```python
from build123d import *

# Parameters (mm, degrees)
SALIENTE_EXTRUIR1_DEPTH = 10
CROQUIS2_R              = 2.5
CORTAR_EXTRUIR1_DEPTH   = 1.5
CROQUIS3_R              = 1.5
CORTAR_EXTRUIR2_DEPTH   = 2
CORTAR_EXTRUIR3_START   = -24
CROQUIS6_R              = 1
CORTAR_EXTRUIR3_DEPTH   = 24
CROQUIS9_W              = 7
CROQUIS9_H              = 5
CROQUIS9_R              = 0.5
SALIENTE_EXTRUIR4_DEPTH = 6
CROQUIS10_W             = 3
CROQUIS10_H             = 3
CORTAR_EXTRUIR4_DEPTH   = 5
REDONDEO1_R             = 5


with BuildPart() as part:
    # Croquis1 → Saliente-Extruir1 (new body)
    with BuildSketch(Plane.XY):
        Polygon((8.5, 0), (-8.5, 0), (-8.5, -12.5), (-12, -12.5), (-12, 2.5), (-12, 15), (-9.5, 15), (-9.5, 2.5), (9.5, 2.5), (9.5, 15), (12, 15), (12, 2.5), (12, -12.5), (8.5, -12.5), align=None)
    extrude(amount=SALIENTE_EXTRUIR1_DEPTH)

    # Croquis2 → Cortar-Extruir1 (cut)
    with BuildSketch(Plane(origin=(-8.5, 0, 0), x_dir=(0, 0, -1), z_dir=(1, 0, 0))):
        with Locations(Location((-5, -8.5, 0), (0, 0, 90))):
            Circle(CROQUIS2_R)
    cortar_extruir1 = extrude(amount=-CORTAR_EXTRUIR1_DEPTH, mode=Mode.SUBTRACT)

    # Croquis3 → Cortar-Extruir2 (cut)
    with BuildSketch(Plane(origin=(-10, 0, 0), x_dir=(0, 0, -1), z_dir=(1, 0, 0))):
        with Locations(Location((-5, -8.5, 0), (0, 0, 90))):
            Circle(CROQUIS3_R)
    cortar_extruir2 = extrude(amount=-CORTAR_EXTRUIR2_DEPTH, mode=Mode.SUBTRACT)

    # Simetría1: Cortar-Extruir1, Cortar-Extruir2 across plane
    add(cortar_extruir1.mirror(Plane(origin=(0, 0, 0), x_dir=(0, 0, 1), z_dir=(1, 0, 0))), mode=Mode.SUBTRACT)
    add(cortar_extruir2.mirror(Plane(origin=(0, 0, 0), x_dir=(0, 0, 1), z_dir=(1, 0, 0))), mode=Mode.SUBTRACT)

    # Croquis6 → Cortar-Extruir3 (cut)
    with BuildSketch(Plane.ZY.offset(12).offset(CORTAR_EXTRUIR3_START)):
        with Locations((5, 12)):
            Circle(CROQUIS6_R)
    extrude(amount=CORTAR_EXTRUIR3_DEPTH, mode=Mode.SUBTRACT)

    # Croquis9 → Saliente-Extruir4 (add)
    with BuildSketch(Plane.ZY.offset(12)):
        with Locations((6.5, 7)):
            Rectangle(CROQUIS9_W, CROQUIS9_H)
        with Locations((5, 7)):
            Circle(CROQUIS9_R, mode=Mode.SUBTRACT)
    extrude(amount=SALIENTE_EXTRUIR4_DEPTH)

    # Croquis10 → Cortar-Extruir4 (cut)
    with BuildSketch(Plane.XZ.offset(-4.5)):
        with Locations((-13.5, 4.5)):
            Rectangle(CROQUIS10_W, CROQUIS10_H)
    extrude(amount=-CORTAR_EXTRUIR4_DEPTH, mode=Mode.SUBTRACT)

    # Redondeo1
    redondeo1_edges = [part.edges().sort_by_distance(p)[0] for p in [
        (10.25, -12.5, 10),
        (-10.25, -12.5, 10),
        (-10.25, -12.5, 0),
        (10.25, -12.5, 0),
        (-10.75, 15, 10),
        (-10.75, 15, 0),
        (10.75, 15, 10),
        (10.75, 15, 0),
    ]]
    fillet(redondeo1_edges, radius=REDONDEO1_R - 0.0001)  # a hair under: the kernel refuses the full size


solid = part.part
```
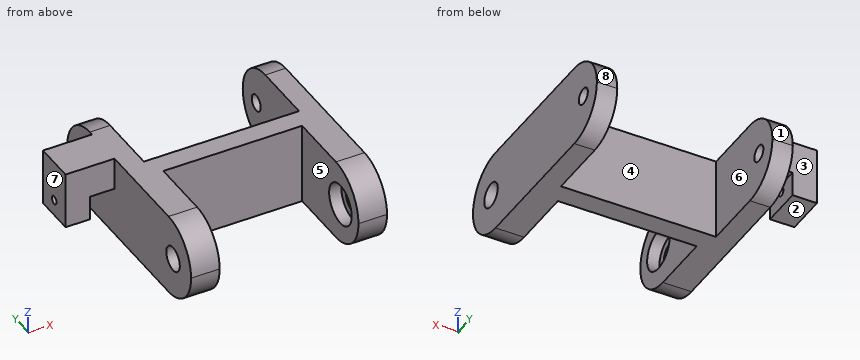
Geometry check sheet. Reference: the model listing, model coordinates, mm. Face numbers are marked on the shaded views. A direction names the side the tool comes from. Give positions to 0.01 mm unless a question says otherwise; leave off trailing zeros. Loops run counter-clockwise (first coordinate to the right, second up) from the corner with the lowest first, then second, coordinate; pieces in that order, holes last. Notation, with made-up numbers: (69.5, 12.25) - (108.5, 12.25) arc R31 ccw to (108.5, 41.25) - close; hole circle Ø5 at (32, 28.25). An arc over 180 degrees is marked (long way). Use CSV: the item, a comma, the result in double quotes. Start each with the question number.
Q1. Section check D-D, the plane y = -8.5. Record the cut outline in (x, z).
Q2. Scan lines: probe 1 along X at (y, z) = (-7.5, 8.5); probe 2 along X at (y, z) = (4.5, 2.25); probe 3 along Y at (x, z) = (-15.5, 8.5). Record each from-to range of solid material in increasing order. Write a range as from..to.
Q3. Section check A-A, the plane y = 7. Record the cut outline in (x, z).
Q4. Section check C-C, the plane x = -16. Record the cut outline in (y, z), and give its area (3 significant figures).
Q5. Release check for a two-part mould opening along X. For the marked faces 6, 7 and 8 record: +X half, -X half, draft (parallel to the pull), parting line (faces both ways), or undercut.
Q6. Section check B-B, the plane y = 3. Record the cut outline in (x, z).
Q7. Access from +Z, -Z, +X, -X, +Y, -Y to the whole of each face (thin tool, end or side, straight path). Record for the marked faces 1, 2, 3, 4 and 5.
Q8. Go/stop test with flat-tipped pins: pin 1 Ø2.5 at (y, z) = (-8.5, 5) entering from +X; pin 2 Ø3.5 at (x, y) = (-14, 7) entering from -Z; pin 3 Ø3 at (x, z) = (-15.5, 7) entering from -Y; pin 4 Ø4 at (y, z) = (-8.5, 5) entering from -X. Record where each tip stops, or that it passes through.
Findings below:
1,outline,"(-12, 0.1) - (-8.5, 0.1) - (-8.5, 2.5) - (-10, 2.5) - (-10, 3.5) - (-12, 3.5) - close; (-12, 6.5) - (-10, 6.5) - (-10, 7.5) - (-8.5, 7.5) - (-8.5, 9.9) - (-12, 9.9) - close; (8.5, 0.1) - (12, 0.1) - (12, 3.5) - (10, 3.5) - (10, 2.5) - (8.5, 2.5) - close; (8.5, 7.5) - (10, 7.5) - (10, 6.5) - (12, 6.5) - (12, 9.9) - (8.5, 9.9) - close"
2,probe 1,"x = -12..-8.5, 8.5..12"
2,probe 2,"x = -12..-9.5, 9.5..12"
2,probe 3,"y = 4.5..9.5"
3,outline,"(-18, 3) - (-15, 3) - (-15, 4.5) - (-18, 4.5) - close; (-18, 5.5) - (-15, 5.5) - (-15, 6) - (-12, 6) - (-12, 0) - (-9.5, 0) - (-9.5, 10) - (-18, 10) - close; (9.5, 0) - (12, 0) - (12, 10) - (9.5, 10) - close"
4,outline,"(4.5, 3) - (9.5, 3) - (9.5, 10) - (4.5, 10) - close; hole circle Ø1 at (7, 5)"
4,area,"34.2 mm^2"
5,face 6,"undercut"
5,face 7,"-X half"
5,face 8,"draft"
6,outline,"(-12, 0) - (-9.5, 0) - (-9.5, 10) - (-12, 10) - close; (9.5, 0) - (12, 0) - (12, 10) - (9.5, 10) - close"
7,face 1,"+Z, +X, -X, +Y"
7,face 2,"-Z, -X, +Y, -Y"
7,face 3,"+Z, -Z, -X, +Y"
7,face 4,"+Z, -Z, +Y"
7,face 5,"+Z, -Z, -Y"
8,pin 1,"passes through"
8,pin 2,"stops at z = 3"
8,pin 3,"stops at y = 4.5"
8,pin 4,"stops at x = -12"
